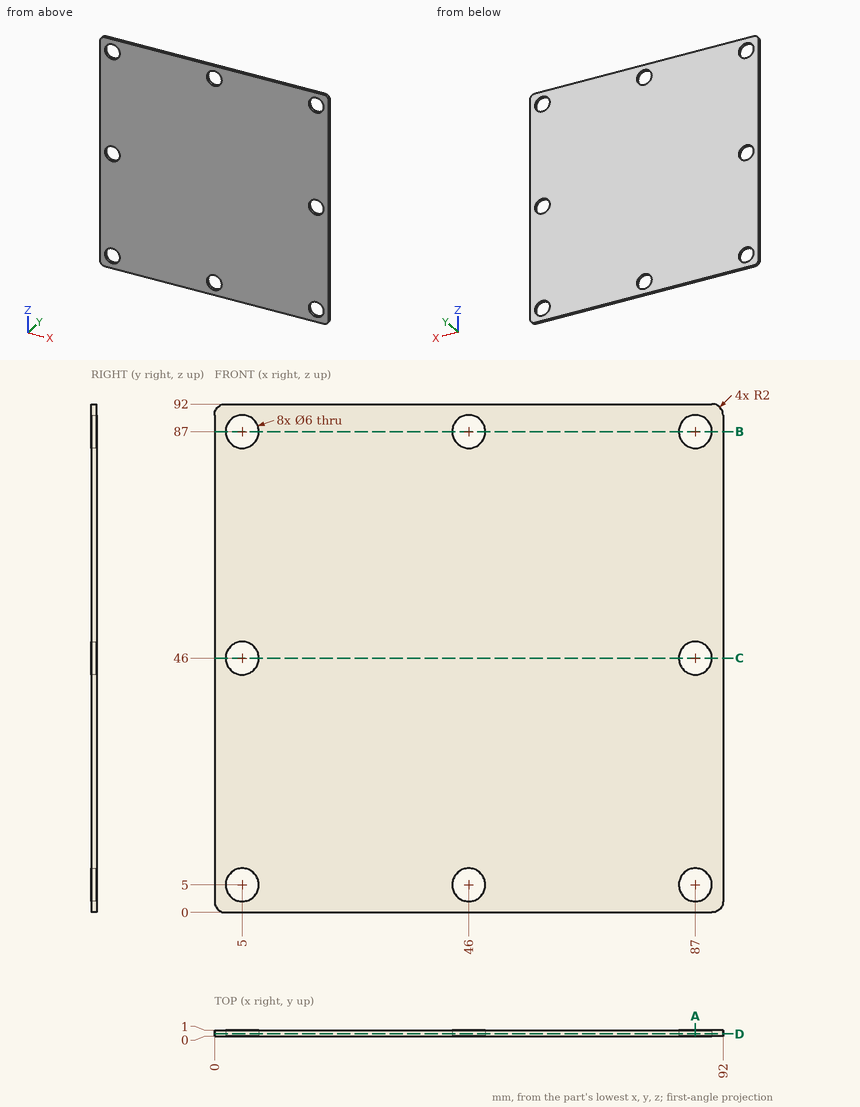
The figure shows three views and two pictorial views of one solid part (mm, origin at its lowest corner). Answer the questions. Round coordinates to 2 decimals unless told otherwise and drop trailing zeros. Loops run counter-clockwise (first coordinate to the right, second up) from the corner with the lowest first, then second, coordinate; pieces in that order, holes last. Notation, with made-up numbers: M 8,-36.75 L 64,-36.75 A18 cw 64,-28.75 Z; hole C 13.5,-27 d9. An arc over 180 degrees is marked long. Return JSON: item names as keys, results as strings.
Q1. This flat-tipped pin is pushed along its axis until it touches: pin 1 Ø3.5 at (x, z) = (5, 46) entering from +Y. Where does it stop, or does it pass through?
Results list:
{"pin 1": "passes through"}
Q2. Find the intervals of material crossed by line 1 along X through (y, z) = (0.8, 87); line 2 along X through (y, z) = (0.3, 46), in increasing order. Write a range as from..to.
Results list:
{"line 1": "x = 0..2, 8..43, 49..84, 90..92", "line 2": "x = 0..2, 8..84, 90..92"}
Q3. Find section B-B, the plane z = 87. Determine the outline of the cut face in (x, y), plus the area to 3 significant figures.
Results list:
{"outline": "M 0,0 L 2,0 L 2,1 L 0,1 Z; M 8,0 L 43,0 L 43,1 L 8,1 Z; M 49,0 L 84,0 L 84,1 L 49,1 Z; M 90,0 L 92,0 L 92,1 L 90,1 Z", "area": "74.0 mm2"}
Q4. Find section C-C, the plane z = 46. Determine the outline of the cut face in (x, y).
Results list:
{"outline": "M 0,0 L 2,0 L 2,1 L 0,1 Z; M 8,0 L 84,0 L 84,1 L 8,1 Z; M 90,0 L 92,0 L 92,1 L 90,1 Z"}
Q5. Find section A-A, the plane x = 87. Determine the outline of the cut face in (y, z), plus the area to 3 significant figures.
Results list:
{"outline": "M 0,0 L 1,0 L 1,2 L 0,2 Z; M 0,8 L 1,8 L 1,43 L 0,43 Z; M 0,49 L 1,49 L 1,84 L 0,84 Z; M 0,90 L 1,90 L 1,92 L 0,92 Z", "area": "74.0 mm2"}
Q6. Find section D-D, the plane y = 0.4. State how many separate pieces and enclosed holes the cut face has, plus the area to 3 significant figures.
Results list:
{"separate pieces": "1", "enclosed holes": "8", "area": "8,230 mm2"}
